```python
from build123d import *

# Parameters (mm, degrees)
SZKIC1_R                    = 14
DODANIE_WYCI_GNI_CIE1_DEPTH = 2
ZAOKR_GLENIE1_R             = 0.4


with BuildPart() as part:
    # Szkic1 → Dodanie-wyciągnięcie1 (new body)
    with BuildSketch(Plane.XY):
        with BuildLine():
            ThreePointArc((-18.639675426, 7.25), (0, -20), (18.639675426, 7.25))
            ThreePointArc((18.639675426, 7.25), (0, 34.5), (-18.639675426, 7.25))
        make_face()
        with Locations((0, 15.5)):
            Circle(SZKIC1_R, mode=Mode.SUBTRACT)
    extrude(amount=DODANIE_WYCI_GNI_CIE1_DEPTH)

    # Zaokrąglenie1
    zaokr_glenie1_edges = [part.edges().sort_by_distance(p)[0] for p in [
        (0, 34.5, 2),
        (-14, 15.5, 2),
        (0, -20, 2),
    ]]
    fillet(zaokr_glenie1_edges, radius=ZAOKR_GLENIE1_R)


solid = part.part
```
Input: part model. Units: mm. Frame: model coordinates. Give positions to 0.01 mm unless a question says otherwise; leave off trailing zeros. Order: outer loops, then holes, each group sorted by start corner. A loop starts at its lowest first (then second) coordinate and runs counter-clockwise, first axis right, second up. Notation, with made-up numbers: M 66.5,62.5 L 125.5,62.5 A9 ccw 125.5,69.5 Z; hole C 38,73 d9. An arc over 180 degrees is marked long. One line per question, with ' | ' between items.
1) Contact query for a flat-ended pin moving along its axis: P1, Ø1, axis at x = -2.5, z = 0.5, coming from the -Y side. Output: stop coordinate, or through.
Filled in:
P1: stops at y = -19.9
2) Section A-A on x = 0. Output: boundary loops of the cut face in (y, z).
Filled in:
outline: M -20,0 L 1.5,0 L 1.5,1.6 A0.4 ccw 1.1,2 L -19.6,2 A0.4 ccw -20,1.6 Z; M 29.5,0 L 34.5,0 L 34.5,1.6 A0.4 ccw 34.1,2 L 29.9,2 A0.4 ccw 29.5,1.6 Z
3) Ray query, L1, parallel to Y at x = 0.5, z = 1; L2, parallel to Y at x = 11, z = 1.2; L3, parallel to X at y = 12, z = 1.1. Return the intervals inside material, ascending.
Filled in:
L1: y = -19.99 to 1.51, 29.49 to 34.49 | L2: y = -16.7 to 6.84, 24.16 to 31.2 | L3: x = -19.84 to -13.56, 13.56 to 19.84
4) Draft query along Y for faces 1 (the face through (-3.03, 1.83, 0.79)), 2 (the face through (-5, 2, 0)). Return one class per face: pulls with the +Y half, pulls with the -Y half, needs draft (parallel to the pull), parting line crosses it, or undercut.
Filled in:
face 1: undercut | face 2: needs draft
5) Section B-B on z = 1.25. Output: boundary loops of the cut face in (x, y).
Filled in:
outline: M -18.64,7.25 A20 ccw long 18.64,7.25 A20 ccw long Z; hole C 0,15.5 d28
